```python
from build123d import *

# Parameters (mm, degrees)
SKETCH1_W           = 165.1
SKETCH1_H           = 101.6
BOSS_EXTRUDE1_DEPTH = 1.905
SKETCH3_R           = 2.667
BOSS_EXTRUDE2_DEPTH = 4.445


with BuildPart() as part:
    # Sketch1 → Boss-Extrude1 (new body)
    with BuildSketch(Plane(origin=(0, 0, 0), x_dir=(1, 0, 0), z_dir=(0, 1, 0))):
        with Locations((82.55, 50.8)):
            Rectangle(SKETCH1_W, SKETCH1_H)
    extrude(amount=BOSS_EXTRUDE1_DEPTH)

    # Sketch3 → Boss-Extrude2 (add)
    with BuildSketch(Plane.XZ):
        with Locations(Location((5.08, -96.52, 0), (0, 0, 270))):
            Circle(SKETCH3_R)
        with Locations(Location((5.08, -5.08, 0), (0, 0, 270))):
            Circle(SKETCH3_R)
        with Locations(Location((160.02, -5.08, 0), (0, 0, 270))):
            Circle(SKETCH3_R)
        with Locations(Location((160.02, -96.52, 0), (0, 0, 270))):
            Circle(SKETCH3_R)
        with Locations(Location((118.11, -83.82, 0), (0, 0, 270))):
            Circle(SKETCH3_R)
        with Locations(Location((60.325, -83.82, 0), (0, 0, 270))):
            Circle(SKETCH3_R)
        with Locations(Location((60.325, -34.925, 0), (0, 0, 270))):
            Circle(SKETCH3_R)
        with Locations(Location((118.11, -34.925, 0), (0, 0, 270))):
            Circle(SKETCH3_R)
    extrude(amount=BOSS_EXTRUDE2_DEPTH)


solid = part.part
```
Build history of the part. All positions in model axes, mm. A direction names the side the tool comes from. Give positions to 0.01 mm unless a question says otherwise; leave off trailing zeros. Loops run counter-clockwise (first coordinate to the right, second up) from the corner with the lowest first, then second, coordinate; pieces in that order, holes last.
1) Band-saw the part on B-B on y = -2. List the corners of the cut face in (x, z) (3 decimals).
Values follow:
outline: circle Ø5.334 at (5.08, -96.52); circle Ø5.334 at (5.08, -5.08); circle Ø5.334 at (60.325, -83.82); circle Ø5.334 at (60.325, -34.925); circle Ø5.334 at (118.11, -83.82); circle Ø5.334 at (118.11, -34.925); circle Ø5.334 at (160.02, -96.52); circle Ø5.334 at (160.02, -5.08)
2) Band-saw the part on C-C on z = -5.08. List the corners of the cut face in (x, y) (3 decimals), then the cut area to 3 significant figures.
Values follow:
outline: (0, 0) - (2.413, 0) - (2.413, -4.445) - (7.747, -4.445) - (7.747, 0) - (157.353, 0) - (157.353, -4.445) - (162.687, -4.445) - (162.687, 0) - (165.1, 0) - (165.1, 1.905) - (0, 1.905) - close
area: 362 mm2
3) Band-saw the part on D-D on z = -47. List the corners of the cut face in (x, y) (3 decimals).
Values follow:
outline: (0, 0) - (165.1, 0) - (165.1, 1.905) - (0, 1.905) - close
4) Two-plate mould, pull along X, no slides. Class faces 3 (the face through (160, -4.445, -5)), 4 (the face through (120.754, -2.191, -83.473)): released by +X, released by -X, zero draft, split by the parting line, or undercut.
Values follow:
face 3: zero draft
face 4: undercut
5) Drop a flat-ended pin along its axis: P1, Ø1.5, axis at x = 62.5, z = -75.5, coming from the -Y side. Give the stop position or say it passes through.
Values follow:
P1: stops at y = 0
6) Probe line 1 along X through (y, z) = (-2.5, -83.5); line 2 along Y through (x, z) = (80.5, -89) (3 decimals); line 3 along X through (y, z) = (-0.5, -84.5). List the from-to ranges inside material, lowest first.
Values follow:
line 1: x = 57.68 to 62.97, 115.46 to 120.76
line 2: y = 0 to 1.905
line 3: x = 57.75 to 62.9, 115.53 to 120.69
7) 3-axis set-ups, long thin cutter, end or side, ignore diameter. For faces 1 (the face through (5, -4.445, -96)), 2 (the face through (157.416, -2.191, -4.502)): which of +Z, -Z, +X, -X, +Y, -Y reach the whole face in a straight line?
Values follow:
face 1: +Z, -Z, +X, -X, -Y
face 2: -Y
8) Band-saw the part on A-A on x = 5.08. List the corners of the cut face in (y, z) (3 decimals), then the cut area to 3 significant figures.
Values follow:
outline: (-4.445, -99.187) - (0, -99.187) - (0, -101.6) - (1.905, -101.6) - (1.905, 0) - (0, 0) - (0, -2.413) - (-4.445, -2.413) - (-4.445, -7.747) - (0, -7.747) - (0, -93.853) - (-4.445, -93.853) - close
area: 241 mm2
